Here's how the part is built. I have some questions about the finished solid (model axes, mm). Face numbers are marked on the shaded views. A direction names the side the tool comes from. Coordinates: 2 decimals unless noted, no trailing zeros. Write each loop counter-clockwise with the first axis right and the second up, starting at its lowest first coordinate (ties: lowest second). Pieces come first, ordered by that corner, then holes. Notation, with made-up numbers: (59, 75) -> (112, 75) arc R12 cw to (112, 80) -> close; hole circle Ø3 at (73.5, 24.25). An arc over 180 degrees is marked (long way). Put each result on its own line as item: value.
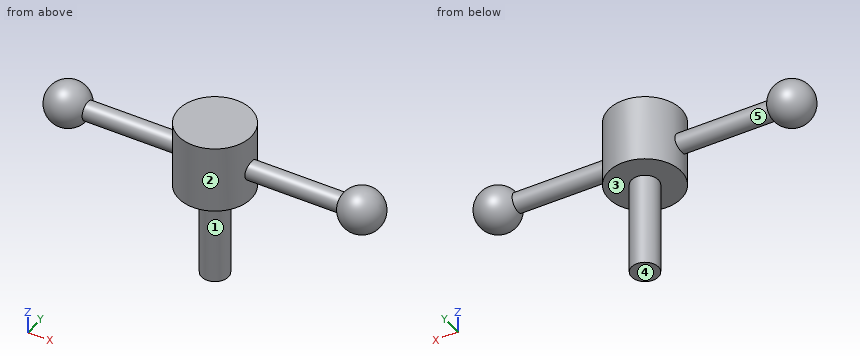
```python
from build123d import *

# Parameters (mm, degrees)
F0_W = 17.1583627141
F0_H = 31.75
F2_W = 6.35
F2_H = 44.45


with BuildPart() as f1:
    # F0 (on Front) → F1 (revolve)
    with BuildSketch(Plane.XZ):
        with Locations((8.579181357, 15.875)):
            Rectangle(F0_W, F0_H)
    revolve(axis=Axis((0, 0, -9.8678829017), (0, 0, -1)))

    # F2 (on Front) → F3 (revolve)
    with BuildSketch(Plane.XZ):
        with Locations((3.175, -22.225)):
            Rectangle(F2_W, F2_H)
    revolve(axis=Axis((0, 0, -33.3453212399), (0, 0, -1)))

    # F4 (on Front) → F5 (revolve)
    with BuildSketch(Plane.XZ):
        with BuildLine():
            Line((-58.4687533851, 14.4232111052), (-7.6910817411, 14.4232111052))
            Line((-7.6910817411, 14.4232111052), (-7.6910817411, 18.8682111052))
            Line((-7.6910817411, 18.8682111052), (-59.4926943332, 18.8682111052))
            ThreePointArc((-59.4926943332, 18.8682111052), (-70.9094594197, 24.3239171398), (-78.7887533851, 14.4232111052))
            Line((-78.7887533851, 14.4232111052), (-58.4687533851, 14.4232111052))
        make_face()
        with BuildLine():
            Line((59.4926943332, 18.8682111052), (7.6910817411, 18.8682111052))
            Line((7.6910817411, 18.8682111052), (7.6910817411, 14.4232111052))
            Line((7.6910817411, 14.4232111052), (78.7887533851, 14.4232111052))
            ThreePointArc((78.7887533851, 14.4232111052), (70.9094594197, 24.3239171398), (59.4926943332, 18.8682111052))
        make_face()
    revolve(axis=Axis((-48.3527202798, 0, 14.4232111052), (-1, 0, 0)))


solid = f1.part
```
Item 1: Imagine slicing it at C-C on z = 12. Write out the boundary of the cut face in (x, y), then the cut area to 3 significant figures.
Output:
outline: (-59.49, -3.73) -> (-16.75, -3.73) arc R17.16 ccw to (16.75, -3.73) -> (59.49, -3.73) arc R9.87 ccw (long way) to (59.49, 3.73) -> (16.75, 3.73) arc R17.16 ccw to (-16.75, 3.73) -> (-59.49, 3.73) arc R9.87 ccw (long way) to start
area: 2,160 mm²
Item 2: For P1, Ø4, axis at x = 2.5, z = -4, coming from the -Y side; P2, Ø8, axis at y = 6, z = -27, coming from the +X side; P3, Ø12, axis at x = -18.5, y = 11.5, coming from the -Z side, each with a flat end and sliding along its axis, tell me the tip position at first contact or that it passes through.
Output:
P1: stops at y = -6.33
P2: stops at x = 6.03
P3: stops at z = 0
Item 3: Imagine slicing it at A-A on x = 0. Write out the boundary of the cut face in (y, z), then the cut area to 3 significant figures.
Output:
outline: (-17.16, 0) -> (-6.35, 0) -> (-6.35, -44.45) -> (6.35, -44.45) -> (6.35, 0) -> (17.16, 0) -> (17.16, 31.75) -> (-17.16, 31.75) -> close
area: 1,650 mm²
Item 4: Which directions (+Z, -Z, +X, -X, +Y, -Y) give clear straight access to the entire face, cutting with the end or side of a thin tool? Please do the marked faces 4 and 5.
Output:
face 4: -Z, +X, -X, +Y, -Y
face 5: none
Item 5: Imagine slicing it at B-B on y = 0. Write out the boundary of the cut face in (x, z).
Output:
outline: (-59.49, 9.98) -> (-17.16, 9.98) -> (-17.16, 0) -> (-6.35, 0) -> (-6.35, -44.45) -> (6.35, -44.45) -> (6.35, 0) -> (17.16, 0) -> (17.16, 9.98) -> (59.49, 9.98) arc R10.16 ccw (long way) to (59.49, 18.87) -> (17.16, 18.87) -> (17.16, 31.75) -> (-17.16, 31.75) -> (-17.16, 18.87) -> (-59.49, 18.87) arc R10.16 ccw (long way) to start
Item 6: If we mould it in two halves opening along X, with no side actions, what happens to the marked faces 1, 2 and 3? For each: released by +X, released by -X, zero draft, split by the parting line, or undercut.
Output:
face 1: split by the parting line
face 2: undercut
face 3: zero draft
Item 7: Please list where these lines run through material, in increasing order: line 1 along Z through (x, y) = (-9, 7.5); line 2 along Y through (x, z) = (-4.5, 23.5); line 3 along Y through (x, z) = (-65.5, 21.5). Write a range as from..to.
Output:
line 1: z = 0..31.75
line 2: y = -16.56..16.56
line 3: y = -6.58..6.58
Item 8: Imagine slicing it at D-D on z = 23. Write out the boundary of the cut face in (x, y).
Output:
outline: circle Ø10.89 at (-68.63, 0); circle Ø34.32 at (0, 0); circle Ø10.89 at (68.63, 0)
